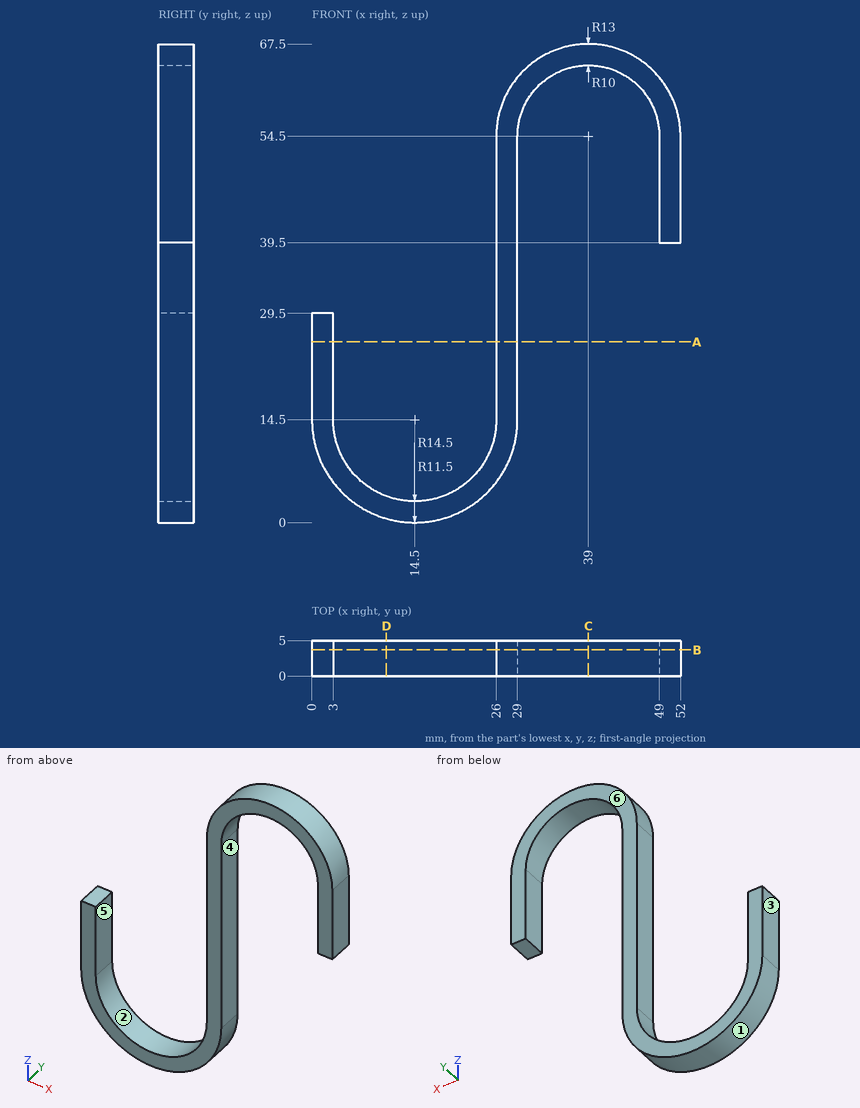
The drawing under review shows one solid part. Ordinate dimensions are in mm from its lowest x, y, z. A direction names the side the tool comes from. Round coordinates to 2 decimals unless told otherwise and drop trailing zeros. Loops run counter-clockwise (first coordinate to the right, second up) from the corner with the lowest first, then second, coordinate; pieces in that order, holes last. Notation, with made-up numbers: (-9.75, 78) - (27.25, 78) arc R19 cw to (27.25, 88) - close; hole circle Ø6 at (62.25, -38.75). An arc over 180 degrees is marked (long way). One line per question, with ' | ' between items.
Q1. Take a section at C-C (x = 39). Give the boundary of the cut face in (y, z), and give its area (3 significant figures).
Taken from the geometry:
outline: (0, 64.5) - (5, 64.5) - (5, 67.5) - (0, 67.5) - close | area: 15.0 mm²
Q2. For line 1 along X through (y, z) = (3.3, 24); line 2 along X through (y, z) = (0.5, 55); line 3 along X through (y, z) = (2.6, 31.5), list the stretches that pass through material, from the lowest coordinate up. Write a range as [from, to].
Taken from the geometry:
line 1: x = [0, 3], [26, 29] | line 2: x = [26.01, 29.01], [48.99, 51.99] | line 3: x = [26, 29]
Q3. Take a section at D-D (x = 10.5). Give the boundary of the cut face in (y, z), and give its area (3 significant figures).
Taken from the geometry:
outline: (0, 0.56) - (5, 0.56) - (5, 3.72) - (0, 3.72) - close | area: 15.8 mm²
Q4. Take a section at B-B (y = 3.7). Give the boundary of the cut face in (x, z).
Taken from the geometry:
outline: (0, 14.5) arc R14.5 ccw to (29, 14.5) - (29, 54.5) arc R10 cw to (49, 54.5) - (49, 39.5) - (52, 39.5) - (52, 54.5) arc R13 ccw to (26, 54.5) - (26, 14.5) arc R11.5 cw to (3, 14.5) - (3, 29.5) - (0, 29.5) - close
Q5. For pin 1 (3 mm diameter, centred on x = 31.5, y = 2, fed in from -Z); pin 2 (1.5 mm diameter, centred on y = 3, z = 49, fed in from -X); pin 3 (2.5 mm diameter, centred on x = 1.5, y = 3, fed in from +Z); pin 4 (8 mm diameter, centred on x = 19, z = 35.5, fed in from -Y), all flat-tipped, find the tip position at first contact; note any pin that passes through.
Taken from the geometry:
pin 1: stops at z = 58.86 | pin 2: stops at x = 26 | pin 3: stops at z = 29.5 | pin 4: passes through
Q6. Take a section at A-A (z = 25.5). Give the boundary of the cut face in (x, y), and give its area (3 significant figures).
Taken from the geometry:
outline: (0, 0) - (3, 0) - (3, 5) - (0, 5) - close; (26, 0) - (29, 0) - (29, 5) - (26, 5) - close | area: 30.0 mm²
Q7. The part is to be moulded in two halves that separate along X. For the marked faces 1, 2 and 3, say which applies: released by +X, released by -X, zero draft, split by the parting line, or undercut.
Taken from the geometry:
face 1: split by the parting line | face 2: undercut | face 3: released by -X
Q8. Tool access review of the marked faces 4, 5 and 6: name each direction out of +Z, -Z, +X, -X, +Y, -Y from which nothing blocks a thin tool from reaching the whole face with its end or side.
Taken from the geometry:
face 4: -Z, +Y, -Y | face 5: +Z, +Y, -Y | face 6: +Z, -Z, +X, -X, +Y
